Check sheet for the modelled part. Datum: model origin and axes. Units: mm. Face numbers are marked on the shaded views. A direction names the side the tool comes from. Round coordinates to 2 decimals unless told otherwise and drop trailing zeros. Order: outer loops, then holes, each group sorted by start corner. A loop starts at its lowest first (then second) coordinate and runs counter-clockwise, first axis right, second up.
Q1. Set-up check for the marked faces 5 and 6: record each of +Z, -Z, +X, -X, +Y, -Y from which the full face is reachable in a straight line by a thin tool's end or side.
Q2. Depth check by flat-ended pin: P1, Ø3, axis at x = 26.5, z = -57.5, coming from the -Y side; P2, Ø2, axis at y = 11, z = -1, coming from the +X side; P3, Ø4.5, axis at x = 17.32, z = -17.32, coming from the -Y side. Enter the tip coordinate at first touch or a pass-through.
Q3. Scan lines: probe 1 along Z at (x, y) = (11.5, 25); probe 2 along Z at (x, y) = (-14.5, -57); probe 3 along Y at (x, z) = (77, 34). Record each from-to range of solid material in increasing order.
Q4. Cross-section at A-A on x = 0. Record the cut outline in (y, z).
Q5. Cross-section at B-B on y = -134. Record the cut outline in (x, z).
Q6. Cross-section at C-C on z = 26.5. Record the cut outline in (x, y), then the cut area to 3 significant figures.
Q7. Cross-section at D-D on x = 57. Record the cut outline in (y, z).
Q8. Mould release check, pull along Z, two halves, no side actions. Record for the marked faces 1, 2, 3 and 4: +Z half, -Z half, draft (parallel to the pull), parting line (faces both ways), or undercut.
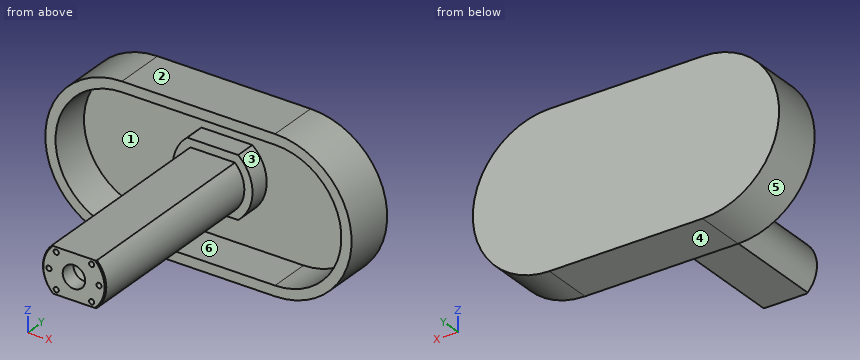
from build123d import *

# Parameters (mm, degrees)
EXTRUDE_1_DEPTH        = 50
CUT_EXTRUDE_1_DEPTH    = 40
EXTRUDE_2_DEPTH        = 20
EXTRUDE_3_DEPTH        = 195
SKETCH_6_R             = 11
CUT_EXTRUDE_2_DEPTH    = 15
SKETCH_7_R             = 18
CUT_EXTRUDE_3_DEPTH    = 200
HOLE_WIZARD_M6_1_D     = 5
HOLE_WIZARD_M6_1_DEPTH = 13
HOLE_WIZARD_M6_1_TIP   = 1.502151548
CHAMFER_1_SIZE         = 1


with BuildPart() as part:
    # 草图1 → 凸台-拉伸1 (new body)
    with BuildSketch(Plane(origin=(0, 0, 0), x_dir=(1, 0, 0), z_dir=(0, 1, 0))):
        with BuildLine():
            Line((-75, 75), (75, 75))
            ThreePointArc((75, 75), (150, 0), (75, -75))
            Line((75, -75), (-75, -75))
            ThreePointArc((-75, -75), (-150, 0), (-75, 75))
        make_face()
    extrude(amount=EXTRUDE_1_DEPTH)

    # 草图2 → 切除-拉伸1 (cut)
    with BuildSketch(Plane.XZ):
        with BuildLine():
            Line((-75, 65), (75, 65))
            ThreePointArc((75, 65), (140, 0), (75, -65))
            Line((75, -65), (-75, -65))
            ThreePointArc((-75, -65), (-140, 0), (-75, 65))
        make_face()
    extrude(amount=-CUT_EXTRUDE_1_DEPTH, mode=Mode.SUBTRACT)

    # 草图4 → 凸台-拉伸2 (add)
    with BuildSketch(Plane.XZ.offset(-40)):
        with BuildLine():
            Line((-24.919871589, 30), (24.919871589, 30))
            ThreePointArc((24.919871589, 30), (39, 0), (24.919871589, -30))
            Line((24.919871589, -30), (-24.919871589, -30))
            ThreePointArc((-24.919871589, -30), (-39, 0), (-24.919871589, 30))
        make_face()
    extrude(amount=EXTRUDE_2_DEPTH)

    # 草图5 → 凸台-拉伸3 (add)
    with BuildSketch(Plane.XZ.offset(-20)):
        with BuildLine():
            Line((-21.840329668, 22), (21.840329668, 22))
            ThreePointArc((21.840329668, 22), (31, 0), (21.840329668, -22))
            Line((21.840329668, -22), (-21.840329668, -22))
            ThreePointArc((-21.840329668, -22), (-31, 0), (-21.840329668, 22))
        make_face()
    extrude(amount=EXTRUDE_3_DEPTH)

    # 草图6 → 切除-拉伸2 (cut)
    with BuildSketch(Plane.XZ.offset(175)):
        with Locations(Location((0, 0, 0), (0, 0, 270))):
            Circle(SKETCH_6_R)
    extrude(amount=-CUT_EXTRUDE_2_DEPTH, mode=Mode.SUBTRACT)

    # 草图7 → 切除-拉伸3 (cut)
    with BuildSketch(Plane(origin=(0, -160, 0), x_dir=(1, 0, 0), z_dir=(0, 1, 0))):
        with Locations(Location((0, 0, 0), (0, 0, 270))):
            Circle(SKETCH_7_R)
    extrude(amount=CUT_EXTRUDE_3_DEPTH, mode=Mode.SUBTRACT)

    # M6 螺纹孔1
    with Locations(Plane(origin=(0, -175, 0), x_dir=(-1, 0, 0), z_dir=(0, -1, 0))):
        with Locations((24.5, 0), (17.324116139, -17.324116139), (-17.324116139, -17.324116139), (-24.5, 0), (-17.324116139, 17.324116139), (17.324116139, 17.324116139)):
            Hole(HOLE_WIZARD_M6_1_D / 2, depth=HOLE_WIZARD_M6_1_DEPTH)
            with Locations((0, 0, -(HOLE_WIZARD_M6_1_DEPTH + HOLE_WIZARD_M6_1_TIP / 2))):  # 118° drill point
                Cone(0, HOLE_WIZARD_M6_1_D / 2, HOLE_WIZARD_M6_1_TIP, mode=Mode.SUBTRACT)

    # 倒角1
    chamfer_1_edges = [part.edges().sort_by_distance(p)[0] for p in [
        (-31, -175, 0),
        (31, -175, 0),
    ]]
    chamfer(chamfer_1_edges, length=CHAMFER_1_SIZE)


solid = part.part
Results found:
1. face 5: -X, +Y, -Y
1. face 6: -Y
2. P1: stops at y = 40
2. P2: stops at x = 150
2. P3: stops at y = -161.85
3. probe 1: z = -75 to -65, -30 to -13.85, 13.85 to 30, 65 to 75
3. probe 2: z = -22 to -10.67, 10.67 to 22
3. probe 3: y = 40 to 50
4. outline: (-175, -22) - (20, -22) - (20, -30) - (40, -30) - (40, -65) - (0, -65) - (0, -75) - (50, -75) - (50, 75) - (0, 75) - (0, 65) - (40, 65) - (40, 30) - (20, 30) - (20, 22) - (-175, 22) - (-175, 11) - (-160, 11) - (-160, 18) - (40, 18) - (40, -18) - (-160, -18) - (-160, -11) - (-175, -11) - close
5. outline: (-21.84, -22) - (21.84, -22) arc R31 ccw to (21.84, 22) - (-21.84, 22) arc R31 ccw to start; hole circle Ø36 at (0, 0)
6. outline: (-145.16, 0) - (-134.35, 0) - (-134.35, 40) - (-28.61, 40) - (-28.61, 20) - (28.61, 20) - (28.61, 40) - (134.35, 40) - (134.35, 0) - (145.16, 0) - (145.16, 50) - (-145.16, 50) - close
6. area: 4,910 mm2
7. outline: (0, -75) - (50, -75) - (50, 75) - (0, 75) - (0, 65) - (40, 65) - (40, -65) - (0, -65) - close
8. face 1: undercut
8. face 2: +Z half
8. face 3: undercut
8. face 4: -Z half
